The model under review builds one solid part; all positions refer to its coordinate system, in mm. Round coordinates to 2 decimals unless told otherwise and drop trailing zeros. Write each loop counter-clockwise with the first axis right and the second up, starting at its lowest first coordinate (ties: lowest second). Pieces come first, ordered by that corner, then holes. Notation, with made-up numbers: (-19.75, 49.5) -> (19.25, 49.5) arc R25 ccw to (19.25, 73.5) -> close; hole circle Ø8 at (70.25, -32.5). An arc over 180 degrees is marked (long way). Answer in a Markdown table with one row per item. Add a question column.
```python
from build123d import *

# Parameters (mm, degrees)
SKETCH2_W            = 285.75
SKETCH2_H            = 6.35
STOCK_DEPTH          = 127
PEDAL_OPENINGS_DEPTH = 6.35
DRILLED_HOLES_REACH  = 8.35
SKETCH5_R            = 3.96875
SKETCH5_R_2          = 3.175


with BuildPart() as part:
    # Sketch2 → Stock (new body)
    with BuildSketch(Plane.XY):
        with Locations((-646.021194965, 51.468778461)):
            Rectangle(SKETCH2_W, SKETCH2_H)
    extrude(amount=-STOCK_DEPTH)

    # Sketch3 → Pedal Openings (cut)
    with BuildSketch(Plane(origin=(0, 54.643778461, 0), x_dir=(1, 0, 0), z_dir=(0, 1, 0))):
        with BuildLine():
            Line((-638.083694965, 69.85), (-653.958694965, 69.85))
            ThreePointArc((-653.958694965, 69.85), (-658.448823025, 67.990128061), (-660.308694965, 63.5))
            Line((-660.308694965, 63.5), (-660.308694965, 0))
            Line((-660.308694965, 0), (-631.733694965, 0))
            Line((-631.733694965, 0), (-631.733694965, 63.5))
            ThreePointArc((-631.733694965, 63.5), (-633.593566904, 67.990128061), (-638.083694965, 69.85))
        make_face()
    extrude(amount=-PEDAL_OPENINGS_DEPTH, mode=Mode.SUBTRACT)

    # Sketch5 → Drilled Holes (cut, up to next)
    with BuildSketch(Plane(origin=(0, 54.643778461, 0), x_dir=(1, 0, 0), z_dir=(0, 1, 0)), mode=Mode.PRIVATE) as drilled_holes_sk1:
        with Locations((-612.683694965, 25.4)):
            Circle(SKETCH5_R)
    drilled_holes_tool1 = extrude(drilled_holes_sk1.sketch, amount=-DRILLED_HOLES_REACH, mode=Mode.PRIVATE) & part.part
    add(drilled_holes_tool1.solids().sort_by_distance((-612.683695, 54.643778, -25.4))[0], mode=Mode.SUBTRACT)
    # Sketch5 → Drilled Holes (cut, up to next)
    with BuildSketch(Plane(origin=(0, 54.643778461, 0), x_dir=(1, 0, 0), z_dir=(0, 1, 0)), mode=Mode.PRIVATE) as drilled_holes_sk2:
        with Locations((-612.683694965, 50.8)):
            Circle(SKETCH5_R)
    drilled_holes_tool2 = extrude(drilled_holes_sk2.sketch, amount=-DRILLED_HOLES_REACH, mode=Mode.PRIVATE) & part.part
    add(drilled_holes_tool2.solids().sort_by_distance((-612.683695, 54.643778, -50.8))[0], mode=Mode.SUBTRACT)
    # Sketch5 → Drilled Holes (cut, up to next)
    with BuildSketch(Plane(origin=(0, 54.643778461, 0), x_dir=(1, 0, 0), z_dir=(0, 1, 0)), mode=Mode.PRIVATE) as drilled_holes_sk3:
        with Locations((-679.358694965, 50.8)):
            Circle(SKETCH5_R)
    drilled_holes_tool3 = extrude(drilled_holes_sk3.sketch, amount=-DRILLED_HOLES_REACH, mode=Mode.PRIVATE) & part.part
    add(drilled_holes_tool3.solids().sort_by_distance((-679.358695, 54.643778, -50.8))[0], mode=Mode.SUBTRACT)
    # Sketch5 → Drilled Holes (cut, up to next)
    with BuildSketch(Plane(origin=(0, 54.643778461, 0), x_dir=(1, 0, 0), z_dir=(0, 1, 0)), mode=Mode.PRIVATE) as drilled_holes_sk4:
        with Locations((-679.358694965, 25.4)):
            Circle(SKETCH5_R)
    drilled_holes_tool4 = extrude(drilled_holes_sk4.sketch, amount=-DRILLED_HOLES_REACH, mode=Mode.PRIVATE) & part.part
    add(drilled_holes_tool4.solids().sort_by_distance((-679.358695, 54.643778, -25.4))[0], mode=Mode.SUBTRACT)
    # Sketch5 → Drilled Holes (cut, up to next)
    with BuildSketch(Plane(origin=(0, 54.643778461, 0), x_dir=(1, 0, 0), z_dir=(0, 1, 0)), mode=Mode.PRIVATE) as drilled_holes_sk5:
        with Locations((-712.061194965, 12.7)):
            Circle(SKETCH5_R)
    drilled_holes_tool5 = extrude(drilled_holes_sk5.sketch, amount=-DRILLED_HOLES_REACH, mode=Mode.PRIVATE) & part.part
    add(drilled_holes_tool5.solids().sort_by_distance((-712.061195, 54.643778, -12.7))[0], mode=Mode.SUBTRACT)
    # Sketch5 → Drilled Holes (cut, up to next)
    with BuildSketch(Plane(origin=(0, 54.643778461, 0), x_dir=(1, 0, 0), z_dir=(0, 1, 0)), mode=Mode.PRIVATE) as drilled_holes_sk6:
        with Locations((-712.061194965, 38.1)):
            Circle(SKETCH5_R)
    drilled_holes_tool6 = extrude(drilled_holes_sk6.sketch, amount=-DRILLED_HOLES_REACH, mode=Mode.PRIVATE) & part.part
    add(drilled_holes_tool6.solids().sort_by_distance((-712.061195, 54.643778, -38.1))[0], mode=Mode.SUBTRACT)
    # Sketch5 → Drilled Holes (cut, up to next)
    with BuildSketch(Plane(origin=(0, 54.643778461, 0), x_dir=(1, 0, 0), z_dir=(0, 1, 0)), mode=Mode.PRIVATE) as drilled_holes_sk7:
        with Locations((-512.671194965, 12.7)):
            Circle(SKETCH5_R)
    drilled_holes_tool7 = extrude(drilled_holes_sk7.sketch, amount=-DRILLED_HOLES_REACH, mode=Mode.PRIVATE) & part.part
    add(drilled_holes_tool7.solids().sort_by_distance((-512.671195, 54.643778, -12.7))[0], mode=Mode.SUBTRACT)
    # Sketch5 → Drilled Holes (cut, up to next)
    with BuildSketch(Plane(origin=(0, 54.643778461, 0), x_dir=(1, 0, 0), z_dir=(0, 1, 0)), mode=Mode.PRIVATE) as drilled_holes_sk8:
        with Locations((-512.671194965, 38.1)):
            Circle(SKETCH5_R)
    drilled_holes_tool8 = extrude(drilled_holes_sk8.sketch, amount=-DRILLED_HOLES_REACH, mode=Mode.PRIVATE) & part.part
    add(drilled_holes_tool8.solids().sort_by_distance((-512.671195, 54.643778, -38.1))[0], mode=Mode.SUBTRACT)
    # Sketch5 → Drilled Holes (cut, up to next)
    with BuildSketch(Plane(origin=(0, 54.643778461, 0), x_dir=(1, 0, 0), z_dir=(0, 1, 0)), mode=Mode.PRIVATE) as drilled_holes_sk9:
        with Locations((-512.671194965, 63.5)):
            Circle(SKETCH5_R)
    drilled_holes_tool9 = extrude(drilled_holes_sk9.sketch, amount=-DRILLED_HOLES_REACH, mode=Mode.PRIVATE) & part.part
    add(drilled_holes_tool9.solids().sort_by_distance((-512.671195, 54.643778, -63.5))[0], mode=Mode.SUBTRACT)
    # Sketch5 → Drilled Holes (cut, up to next)
    with BuildSketch(Plane(origin=(0, 54.643778461, 0), x_dir=(1, 0, 0), z_dir=(0, 1, 0)), mode=Mode.PRIVATE) as drilled_holes_sk10:
        with Locations((-512.671194965, 88.9)):
            Circle(SKETCH5_R)
    drilled_holes_tool10 = extrude(drilled_holes_sk10.sketch, amount=-DRILLED_HOLES_REACH, mode=Mode.PRIVATE) & part.part
    add(drilled_holes_tool10.solids().sort_by_distance((-512.671195, 54.643778, -88.9))[0], mode=Mode.SUBTRACT)
    # Sketch5 → Drilled Holes (cut, up to next)
    with BuildSketch(Plane(origin=(0, 54.643778461, 0), x_dir=(1, 0, 0), z_dir=(0, 1, 0)), mode=Mode.PRIVATE) as drilled_holes_sk11:
        with Locations((-512.671194965, 114.3)):
            Circle(SKETCH5_R)
    drilled_holes_tool11 = extrude(drilled_holes_sk11.sketch, amount=-DRILLED_HOLES_REACH, mode=Mode.PRIVATE) & part.part
    add(drilled_holes_tool11.solids().sort_by_distance((-512.671195, 54.643778, -114.3))[0], mode=Mode.SUBTRACT)
    # Sketch5 → Drilled Holes (cut, up to next)
    with BuildSketch(Plane(origin=(0, 54.643778461, 0), x_dir=(1, 0, 0), z_dir=(0, 1, 0)), mode=Mode.PRIVATE) as drilled_holes_sk12:
        with Locations((-779.371194965, 88.9)):
            Circle(SKETCH5_R)
    drilled_holes_tool12 = extrude(drilled_holes_sk12.sketch, amount=-DRILLED_HOLES_REACH, mode=Mode.PRIVATE) & part.part
    add(drilled_holes_tool12.solids().sort_by_distance((-779.371195, 54.643778, -88.9))[0], mode=Mode.SUBTRACT)
    # Sketch5 → Drilled Holes (cut, up to next)
    with BuildSketch(Plane(origin=(0, 54.643778461, 0), x_dir=(1, 0, 0), z_dir=(0, 1, 0)), mode=Mode.PRIVATE) as drilled_holes_sk13:
        with Locations((-779.371194965, 114.3)):
            Circle(SKETCH5_R)
    drilled_holes_tool13 = extrude(drilled_holes_sk13.sketch, amount=-DRILLED_HOLES_REACH, mode=Mode.PRIVATE) & part.part
    add(drilled_holes_tool13.solids().sort_by_distance((-779.371195, 54.643778, -114.3))[0], mode=Mode.SUBTRACT)
    # Sketch5 → Drilled Holes (cut, up to next)
    with BuildSketch(Plane(origin=(0, 54.643778461, 0), x_dir=(1, 0, 0), z_dir=(0, 1, 0)), mode=Mode.PRIVATE) as drilled_holes_sk14:
        with Locations((-779.371194965, 63.5)):
            Circle(SKETCH5_R)
    drilled_holes_tool14 = extrude(drilled_holes_sk14.sketch, amount=-DRILLED_HOLES_REACH, mode=Mode.PRIVATE) & part.part
    add(drilled_holes_tool14.solids().sort_by_distance((-779.371195, 54.643778, -63.5))[0], mode=Mode.SUBTRACT)
    # Sketch5 → Drilled Holes (cut, up to next)
    with BuildSketch(Plane(origin=(0, 54.643778461, 0), x_dir=(1, 0, 0), z_dir=(0, 1, 0)), mode=Mode.PRIVATE) as drilled_holes_sk15:
        with Locations((-779.371194965, 38.1)):
            Circle(SKETCH5_R)
    drilled_holes_tool15 = extrude(drilled_holes_sk15.sketch, amount=-DRILLED_HOLES_REACH, mode=Mode.PRIVATE) & part.part
    add(drilled_holes_tool15.solids().sort_by_distance((-779.371195, 54.643778, -38.1))[0], mode=Mode.SUBTRACT)
    # Sketch5 → Drilled Holes (cut, up to next)
    with BuildSketch(Plane(origin=(0, 54.643778461, 0), x_dir=(1, 0, 0), z_dir=(0, 1, 0)), mode=Mode.PRIVATE) as drilled_holes_sk16:
        with Locations((-779.371194965, 12.7)):
            Circle(SKETCH5_R)
    drilled_holes_tool16 = extrude(drilled_holes_sk16.sketch, amount=-DRILLED_HOLES_REACH, mode=Mode.PRIVATE) & part.part
    add(drilled_holes_tool16.solids().sort_by_distance((-779.371195, 54.643778, -12.7))[0], mode=Mode.SUBTRACT)
    # Sketch5 → Drilled Holes (cut, up to next)
    with BuildSketch(Plane(origin=(0, 54.643778461, 0), x_dir=(1, 0, 0), z_dir=(0, 1, 0)), mode=Mode.PRIVATE) as drilled_holes_sk17:
        with Locations((-576.171194965, 73.025)):
            Circle(SKETCH5_R)
    drilled_holes_tool17 = extrude(drilled_holes_sk17.sketch, amount=-DRILLED_HOLES_REACH, mode=Mode.PRIVATE) & part.part
    add(drilled_holes_tool17.solids().sort_by_distance((-576.171195, 54.643778, -73.025))[0], mode=Mode.SUBTRACT)
    # Sketch5 → Drilled Holes (cut, up to next)
    with BuildSketch(Plane(origin=(0, 54.643778461, 0), x_dir=(1, 0, 0), z_dir=(0, 1, 0)), mode=Mode.PRIVATE) as drilled_holes_sk18:
        with Locations((-576.171194965, 111.125)):
            Circle(SKETCH5_R)
    drilled_holes_tool18 = extrude(drilled_holes_sk18.sketch, amount=-DRILLED_HOLES_REACH, mode=Mode.PRIVATE) & part.part
    add(drilled_holes_tool18.solids().sort_by_distance((-576.171195, 54.643778, -111.125))[0], mode=Mode.SUBTRACT)
    # Sketch5 → Drilled Holes (cut, up to next)
    with BuildSketch(Plane(origin=(0, 54.643778461, 0), x_dir=(1, 0, 0), z_dir=(0, 1, 0)), mode=Mode.PRIVATE) as drilled_holes_sk19:
        with Locations((-715.871194965, 111.125)):
            Circle(SKETCH5_R)
    drilled_holes_tool19 = extrude(drilled_holes_sk19.sketch, amount=-DRILLED_HOLES_REACH, mode=Mode.PRIVATE) & part.part
    add(drilled_holes_tool19.solids().sort_by_distance((-715.871195, 54.643778, -111.125))[0], mode=Mode.SUBTRACT)
    # Sketch5 → Drilled Holes (cut, up to next)
    with BuildSketch(Plane(origin=(0, 54.643778461, 0), x_dir=(1, 0, 0), z_dir=(0, 1, 0)), mode=Mode.PRIVATE) as drilled_holes_sk20:
        with Locations((-715.871194965, 73.025)):
            Circle(SKETCH5_R)
    drilled_holes_tool20 = extrude(drilled_holes_sk20.sketch, amount=-DRILLED_HOLES_REACH, mode=Mode.PRIVATE) & part.part
    add(drilled_holes_tool20.solids().sort_by_distance((-715.871195, 54.643778, -73.025))[0], mode=Mode.SUBTRACT)
    # Sketch5 → Drilled Holes (cut, up to next)
    with BuildSketch(Plane(origin=(0, 54.643778461, 0), x_dir=(1, 0, 0), z_dir=(0, 1, 0)), mode=Mode.PRIVATE) as drilled_holes_sk21:
        with Locations((-754.764944965, 76.2)):
            Circle(SKETCH5_R_2)
    drilled_holes_tool21 = extrude(drilled_holes_sk21.sketch, amount=-DRILLED_HOLES_REACH, mode=Mode.PRIVATE) & part.part
    add(drilled_holes_tool21.solids().sort_by_distance((-754.764945, 54.643778, -76.2))[0], mode=Mode.SUBTRACT)
    # Sketch5 → Drilled Holes (cut, up to next)
    with BuildSketch(Plane(origin=(0, 54.643778461, 0), x_dir=(1, 0, 0), z_dir=(0, 1, 0)), mode=Mode.PRIVATE) as drilled_holes_sk22:
        with Locations((-743.334944965, 76.2)):
            Circle(SKETCH5_R_2)
    drilled_holes_tool22 = extrude(drilled_holes_sk22.sketch, amount=-DRILLED_HOLES_REACH, mode=Mode.PRIVATE) & part.part
    add(drilled_holes_tool22.solids().sort_by_distance((-743.334945, 54.643778, -76.2))[0], mode=Mode.SUBTRACT)
    # Sketch5 → Drilled Holes (cut, up to next)
    with BuildSketch(Plane(origin=(0, 54.643778461, 0), x_dir=(1, 0, 0), z_dir=(0, 1, 0)), mode=Mode.PRIVATE) as drilled_holes_sk23:
        with Locations((-636.178694965, 79.375)):
            Circle(SKETCH5_R_2)
    drilled_holes_tool23 = extrude(drilled_holes_sk23.sketch, amount=-DRILLED_HOLES_REACH, mode=Mode.PRIVATE) & part.part
    add(drilled_holes_tool23.solids().sort_by_distance((-636.178695, 54.643778, -79.375))[0], mode=Mode.SUBTRACT)
    # Sketch5 → Drilled Holes (cut, up to next)
    with BuildSketch(Plane(origin=(0, 54.643778461, 0), x_dir=(1, 0, 0), z_dir=(0, 1, 0)), mode=Mode.PRIVATE) as drilled_holes_sk24:
        with Locations((-623.478694965, 79.375)):
            Circle(SKETCH5_R_2)
    drilled_holes_tool24 = extrude(drilled_holes_sk24.sketch, amount=-DRILLED_HOLES_REACH, mode=Mode.PRIVATE) & part.part
    add(drilled_holes_tool24.solids().sort_by_distance((-623.478695, 54.643778, -79.375))[0], mode=Mode.SUBTRACT)


solid = part.part
```
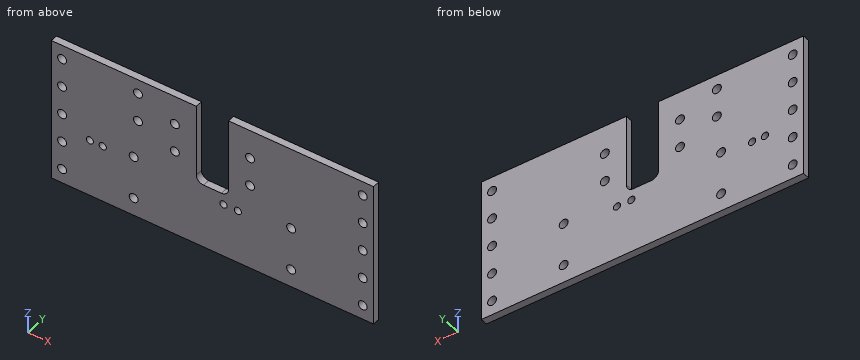
1. For L1, parallel to X at y = 53, z = -25.4; L2, parallel to X at y = 51.25, z = -51.5; L3, parallel to X at y = 49.75, z = -80, list the stretches that pass through material, from the lowest coordinate up.
2. Add section B-B on z = -12.7. Write out the cut boundary in (x, y).
3. Add section A-A on z = -88.9. Write out the cut boundary in (x, y).
4. Add section C-C on y = 50.5. State how many separate pieces and enclosed holes the cut face has, plus the area to 3 significant figures.
5. Insertion check: pin 1 Ø7 at (x, z) = (-679.36, -50.8) entering from -Y. The pin has a flat end and moves straight along its axis. Give the tip position at first contact, or say it passes through.
Filled in:
| question | item | result |
|---|---|---|
| 1 | L1 | -788.9 to -683.33, -675.39 to -660.31, -631.73 to -616.65, -608.71 to -503.15 |
| 1 | L2 | -788.9 to -683.27, -675.45 to -660.31, -631.73 to -616.59, -608.78 to -503.15 |
| 1 | L3 | -788.9 to -639.29, -633.07 to -626.59, -620.37 to -503.15 |
| 2 | outline | (-788.9, 48.29) -> (-783.34, 48.29) -> (-783.34, 54.64) -> (-788.9, 54.64) -> close; (-775.4, 48.29) -> (-716.03, 48.29) -> (-716.03, 54.64) -> (-775.4, 54.64) -> close; (-708.09, 48.29) -> (-660.31, 48.29) -> (-660.31, 54.64) -> (-708.09, 54.64) -> close; (-631.73, 48.29) -> (-516.64, 48.29) -> (-516.64, 54.64) -> (-631.73, 54.64) -> close; (-508.7, 48.29) -> (-503.15, 48.29) -> (-503.15, 54.64) -> (-508.7, 54.64) -> close |
| 3 | outline | (-788.9, 48.29) -> (-783.34, 48.29) -> (-783.34, 54.64) -> (-788.9, 54.64) -> close; (-775.4, 48.29) -> (-516.64, 48.29) -> (-516.64, 54.64) -> (-775.4, 54.64) -> close; (-508.7, 48.29) -> (-503.15, 48.29) -> (-503.15, 54.64) -> (-508.7, 54.64) -> close |
| 4 | separate pieces | 1 |
| 4 | enclosed holes | 24 |
| 4 | area | 33,200 mm² |
| 5 | pin 1 | through |
